Source: CAD feature listing. Evaluate the final solid. Frame: model axes, mm. A direction names the side the tool comes from. Give positions to 0.01 mm unless a question says otherwise; leave off trailing zeros. Write each loop counter-clockwise with the first axis right and the second up, starting at its lowest first coordinate (ties: lowest second). Pieces come first, ordered by that corner, then holes. Notation, with made-up numbers: (40, 71.25) -> (84, 71.25) arc R29 cw to (84, 99.25) -> close; hole circle Ø7 at (52.5, -26). An arc over 180 degrees is marked (long way). Use one line per item in the form item = value. Start each with the question number.
(1) Cut plane D-D, the plane z = -14. Output: boundary loops of the cut face in (x, y), and give its area (3 significant figures).
(2) Set-up query: faces 1 (the face through (-3, -1, -16.5)), 2 (the face through (-2.54, -3.56, -15.51)), 3 (the face through (-5, 1, -8)). Return all of +Z, -Z, +X, -X, +Y, -Y with unobstructed straight access to the full face (end or side cutting, diameter ignored); none if empty.
(3) Draft query along Y for faces 4 (the face through (-3, -2.55, -16)), 5 (the face through (0, 1, -8)), 6 (the face through (-2, 2, -8)), 7 (the face through (-3, -4.55, -17)). Return one class per face: pulls with the +Y half, pulls with the -Y half, needs draft (parallel to the pull), parting line crosses it, or undercut.
(4) Cut plane A-A, the plane y = -1. Output: boundary loops of the cut face in (x, z), and give its area (3 significant figures).
(5) Cut plane C-C, the plane x = -3.8. Output: boundary loops of the cut face in (y, z).
(6) Material intervals for line 1 along Z through (x, y) = (-2.3, -2.5); line 2 along Y through (x, z) = (-4.2, -3); line 3 along Z through (x, y) = (-4.3, -3.25), sorted ascending. Write a range as from..to.
(7) Cut plane B-B, the plane z = -1.75. Output: boundary loops of the cut face in (x, y).
(8) First-contact query: P1, Ø1, axis at x = -3, z = -9.5, coming from the -Y side. Flat tip, straight axial feed; report the tip coordinate or a pass-through.
Autodesk Inventor part; units mm, degrees
ref_plane "YZ Plane" through (0, 0, 0) normal (1, 0, 0) x (0, 1, 0)
ref_plane "XZ Plane" through (0, 0, 0) normal (0, 1, 0) x (-1, 0, 0)
ref_plane "XY Plane" through (0, 0, 0) normal (0, 0, 1) x (1, 0, 0)
sketch "Эскиз1" plane through (0, 0, 0) normal (0, 1, 0) x (-1, 0, 0)
  line L0 (0, 0) -> (5, 0)
  line L1 (5, 0) -> (5, -8.25)
  line L2 (5, -8.25) -> (0, -8.25)
  line L3 (0, -8.25) -> (0, 0)
  dimension "d0" = 5
  dimension "d1" = 8.25
extrude "Выдавливание1" add sketch "Эскиз1" along normal blind 2
sketch "Эскиз2" plane through (-5, 0, -8.25) normal (-1, 0, 0) x (0, 0, 1)
  line L0 (8.25, 2) -> (0, 2)
  line L1 (8.25, 2) -> (10.25, 2)
  line L2 (10.25, 2) -> (10.25, -4.55)
  line L3 (10.25, -4.55) -> (8.25, -4.55)
  line L4 (8.25, -4.55) -> (8.25, 2)
  line L5 (8.25, -4.55) -> (6.25, -4.55)
  line L6 (6.25, -4.55) -> (6.25, -2.55)
  line L7 (6.25, -2.55) -> (8.25, -2.55)
  line L8 (8.25, -2.55) -> (8.25, -4.55)
  line L9 (6.25, -2.55) -> (8.25, -4.55)
  point P0 (8.25, 0)
  dimension "d4" = 2
  dimension "d5" = 6.55
  dimension "d6" = 2
  dimension "d7" = 2
extrude "Выдавливание2" add sketch "Эскиз2" against normal blind 5 contours L1 L2 L3 L4 | L4 L9 L7
mirror "Зеркальное отражение1" about plane through (0, 0, -8.25) normal (0, 0, -1)
properties part number "Тестовая крышка"
Geometry says:
q1.outline = (-5, 0) -> (0, 0) -> (0, 2) -> (-5, 2) -> close
q1.area = 10.0 mm^2
q2.face_1 = +X, -X
q2.face_2 = +X, -X, -Y
q2.face_3 = +Z, -Z, -X, +Y, -Y
q3.face_4 = undercut
q3.face_5 = needs draft
q3.face_6 = pulls with the +Y half
q3.face_7 = pulls with the -Y half
q4.outline = (-5, -18.5) -> (0, -18.5) -> (0, -16.5) -> (-5, -16.5) -> close; (-5, 0) -> (0, 0) -> (0, 2) -> (-5, 2) -> close
q4.area = 20.0 mm^2
q5.outline = (-4.55, -18.5) -> (2, -18.5) -> (2, 2) -> (-4.55, 2) -> (-4.55, 0) -> (-2.55, -2) -> (-2.55, 0) -> (0, 0) -> (0, -16.5) -> (-2.55, -16.5) -> (-2.55, -14.5) -> (-4.55, -16.5) -> close
q6.line_1 = -18.5..-16.5, 0..2
q6.line_2 = 0..2
q6.line_3 = -18.5..-15.2, -1.3..2
q7.outline = (-5, -2.8) -> (0, -2.8) -> (0, -2.55) -> (-5, -2.55) -> close; (-5, 0) -> (0, 0) -> (0, 2) -> (-5, 2) -> close
q8.P1 = 0
